```python
from build123d import *

# Parameters (mm, degrees)
SKETCH1_W           = 46
SKETCH1_H           = 160
SKETCH1_R           = 3.05
SKETCH1_R_2         = 4.425
BOSS_EXTRUDE2_DEPTH = 5
SKETCH4_W           = 46
SKETCH4_H           = 160
BOSS_EXTRUDE3_DEPTH = 5
SKETCH5_R           = 16.5
CUT_EXTRUDE2_DEPTH  = 5
SKETCH5_6_R         = 20.5
SKETCH5_6_R_2       = 16.5
BOSS_EXTRUDE5_DEPTH = 10
BOSS_EXTRUDE7_DEPTH = 61.5
SKETCH8_W           = 11.5
SKETCH8_H           = 67.35
SKETCH8_H_2         = 92.65
CUT_EXTRUDE3_DEPTH  = 10
SKETCH10_W          = 11.5
SKETCH10_H          = 115.012630191
CUT_EXTRUDE5_DEPTH  = 10
SKETCH11_R          = 4.425
CUT_EXTRUDE6_DEPTH  = 10
SKETCH12_W          = 11.5
SKETCH12_H          = 11.545
CUT_EXTRUDE7_DEPTH  = 10
SKETCH13_W          = 11.5
SKETCH13_H          = 11.545
CUT_EXTRUDE8_DEPTH  = 10


with BuildPart() as part:
    # Sketch1 → Boss-Extrude2 (new body)
    with BuildSketch(Plane(origin=(0, 0, 0), x_dir=(1, 0, 0), z_dir=(0, 1, 0))):
        with Locations((0, -55)):
            Rectangle(SKETCH1_W, SKETCH1_H)
        with Locations(Location((0, 0, 0), (0, 0, 270))):
            Circle(SKETCH1_R, mode=Mode.SUBTRACT)
        with Locations(Location((0, -113.03, 0), (0, 0, 270))):
            Circle(SKETCH1_R_2, mode=Mode.SUBTRACT)
    extrude(amount=BOSS_EXTRUDE2_DEPTH)



with BuildPart() as body_2:
    # Sketch4 → Boss-Extrude3 (new body)
    with BuildSketch(Plane(origin=(0, 71.5, 0), x_dir=(1, 0, 0), z_dir=(0, 1, 0))):
        with Locations((0, -55)):
            Rectangle(SKETCH4_W, SKETCH4_H)
    extrude(amount=-BOSS_EXTRUDE3_DEPTH)

    # Sketch5 → Cut-Extrude2 (cut)
    with BuildSketch(Plane(origin=(0, 71.5, 0), x_dir=(1, 0, 0), z_dir=(0, 1, 0))):
        with Locations(Location((0, 0, 0), (0, 0, 270))):
            Circle(SKETCH5_R)
    extrude(amount=-CUT_EXTRUDE2_DEPTH, mode=Mode.SUBTRACT)

    # Sketch5<6> → Boss-Extrude5 (add)
    with BuildSketch(Plane(origin=(0, 71.5, 0), x_dir=(1, 0, 0), z_dir=(0, 1, 0))):
        with Locations(Location((0, 0, 0), (0, 0, 90))):
            Circle(SKETCH5_6_R)
        with Locations(Location((0, 0, 0), (0, 0, 270))):
            Circle(SKETCH5_6_R_2, mode=Mode.SUBTRACT)
    extrude(amount=BOSS_EXTRUDE5_DEPTH)


with BuildPart() as part_1:
    add(part.part)

    add(body_2.part)  # Boss-Extrude7 merges body 2
    # Sketch7 → Boss-Extrude7 (add)
    with BuildSketch(Plane(origin=(0, 5, 0), x_dir=(1, 0, 0), z_dir=(0, 1, 0))):
        with BuildLine():
            Line((7.5, -57.65), (-7.5, -57.65))
            Line((-7.5, -57.65), (-7.5, -62.65))
            Line((-7.5, -62.65), (-3, -62.65))
            ThreePointArc((-3, -62.65), (0, -59.65), (3, -62.65))
            Line((3, -62.65), (7.5, -62.65))
            Line((7.5, -62.65), (7.5, -57.65))
        make_face()
        with BuildLine():
            Line((-3, -62.65), (-7.5, -62.65))
            Line((-7.5, -62.65), (-7.5, -67.65))
            Line((-7.5, -67.65), (7.5, -67.65))
            Line((7.5, -67.65), (7.5, -62.65))
            Line((7.5, -62.65), (3, -62.65))
            ThreePointArc((3, -62.65), (0, -65.65), (-3, -62.65))
        make_face()
        with BuildLine():
            ThreePointArc((3, -62.65), (0, -59.65), (-3, -62.65))
            Line((-3, -62.65), (3, -62.65))
        make_face()
        with BuildLine():
            Line((3, -62.65), (-3, -62.65))
            ThreePointArc((-3, -62.65), (0, -65.65), (3, -62.65))
        make_face()
    extrude(amount=BOSS_EXTRUDE7_DEPTH)

    # Sketch8 → Cut-Extrude3 (cut)
    with BuildSketch(Plane(origin=(0, 5, 0), x_dir=(1, 0, 0), z_dir=(0, 1, 0))):
        with Locations((-17.25, -101.325)):
            Rectangle(SKETCH8_W, SKETCH8_H)
        with Locations((-17.25, -21.325)):
            Rectangle(SKETCH8_W, SKETCH8_H_2)
        with Locations((17.25, -101.325)):
            Rectangle(SKETCH8_W, SKETCH8_H)
        with Locations((17.25, -21.325)):
            Rectangle(SKETCH8_W, SKETCH8_H_2)
    extrude(amount=-CUT_EXTRUDE3_DEPTH, mode=Mode.SUBTRACT)

    # Sketch10 → Cut-Extrude5 (cut)
    with BuildSketch(Plane.XZ.offset(-66.5)):
        with Locations((-17.25, 77.493684905)):
            Rectangle(SKETCH10_W, SKETCH10_H)
        with Locations((17.25, 77.493684905)):
            Rectangle(SKETCH10_W, SKETCH10_H)
    extrude(amount=-CUT_EXTRUDE5_DEPTH, mode=Mode.SUBTRACT)

    # Sketch11 → Cut-Extrude6 (cut)
    with BuildSketch(Plane.XZ.offset(-66.5)):
        with Locations(Location((0, 113.03, 0), (0, 0, 90))):
            Circle(SKETCH11_R)
    extrude(amount=-CUT_EXTRUDE6_DEPTH, mode=Mode.SUBTRACT)

    # Sketch12 → Cut-Extrude7 (cut)
    with BuildSketch(Plane(origin=(0, 5, 0), x_dir=(1, 0, 0), z_dir=(0, 1, 0))):
        with Locations((-5.75, -129.2275)):
            Rectangle(SKETCH12_W, SKETCH12_H)
        with Locations((5.75, -129.2275)):
            Rectangle(SKETCH12_W, SKETCH12_H)
    extrude(amount=-CUT_EXTRUDE7_DEPTH, mode=Mode.SUBTRACT)

    # Sketch13 → Cut-Extrude8 (cut)
    with BuildSketch(Plane(origin=(0, 71.5, 0), x_dir=(1, 0, 0), z_dir=(0, 1, 0))):
        with Locations((-5.75, -129.2275)):
            Rectangle(SKETCH13_W, SKETCH13_H)
        with Locations((5.75, -129.2275)):
            Rectangle(SKETCH13_W, SKETCH13_H)
    extrude(amount=-CUT_EXTRUDE8_DEPTH, mode=Mode.SUBTRACT)


solid = part_1.part
```
Geometry check sheet. Reference: the model listing, model coordinates, mm. A direction names the side the tool comes from. Round coordinates to 2 decimals unless told otherwise and drop trailing zeros. Loops run counter-clockwise (first coordinate to the right, second up) from the corner with the lowest first, then second, coordinate; pieces in that order, holes last. Notation, with made-up numbers: (22.5, -31) - (46.5, -31) arc R14 ccw to (46.5, -4) - close; hole circle Ø8 at (-32, 62.25). An arc over 180 degrees is marked (long way). Use a Markdown table: item, result.
Q1. Access from +Z, -Z, +X, -X, +Y, -Y to the whole of each face (thin tool, end or side, straight path). Record for faces 5 (the flat face through (7.5, 35, 63)), 6 (the flat face through (-11.5, 3, 50)), 7 (the flat face through (-7.5, 35, 63)), 8 (the flat face through (0, 35, 57.65)).
Solutions:
| item | result |
|---|---|
| face 5 | +Z, -Z, +X |
| face 6 | +Z, -Z, -X, -Y |
| face 7 | +Z, -Z, -X |
| face 8 | -Z, +X, -X |
Q2. Material ranges on line 1 (Y direction, x = 5, z = 46); line 2 (X direction, y = 1.9, z = 0); line 3 (X direction, y = 2, z = 113), recorded low to high.
Solutions:
| item | result |
|---|---|
| line 1 | y = 0 to 5, 66.5 to 71.5 |
| line 2 | x = -11.5 to -3.05, 3.05 to 11.5 |
| line 3 | x = -11.5 to -4.42, 4.42 to 11.5 |
Q3. Cross-section at B-B on x = 0. State how many separate pieces and enclosed holes the cut face has, plus the area to 3 significant figures.
Solutions:
| item | result |
|---|---|
| separate pieces | 5 |
| enclosed holes | 0 |
| area | 1,900 mm2 |
Q4. Go/stop test with flat-tipped pins: P1, Ø2.5, axis at x = -18, y = 69, coming from the +Z side; P2, Ø4, axis at x = 9, z = 21.5, coming from the +Y side; P3, Ø2, axis at x = 6, z = 28, coming from the -Y side; P4, Ø4, axis at y = 69.5, z = 81.5, coming from the +X side. Record where each tip stops, or that it passes through.
Solutions:
| item | result |
|---|---|
| P1 | stops at z = 19.99 |
| P2 | stops at y = 71.5 |
| P3 | stops at y = 0 |
| P4 | stops at x = 11.5 |
Q5. Draft check along Z on faces 1 (the cylindrical face through (-1.33, 68.96, 117.25)), 2 (the flat face through (11.5, 3, 48)), 3 (the flat face through (0, 2, -25)), 4 (the flat face through (0, 35, 67.65)). Enter one of: released by +Z, released by -Z, zero draft, split by the parting line, or undercut.
Solutions:
| item | result |
|---|---|
| face 1 | undercut |
| face 2 | zero draft |
| face 3 | released by -Z |
| face 4 | released by +Z |
Q6. Cross-section at C-C on z = 14.5. Record the cut outline in (x, y), plus the area to 3 significant figures.
Solutions:
| item | result |
|---|---|
| outline | (-23, 66.5) - (-7.87, 66.5) - (-7.87, 81.5) - (-14.49, 81.5) - (-14.49, 71.5) - (-23, 71.5) - close; (-11.5, 0) - (11.5, 0) - (11.5, 5) - (-11.5, 5) - close; (7.87, 66.5) - (23, 66.5) - (23, 71.5) - (14.49, 71.5) - (14.49, 81.5) - (7.87, 81.5) - close |
| area | 399 mm2 |
Q7. Cross-section at A-A on z = 113.03. Record the cut outline in (x, y) (3 decimals), plus the area to 4 significant figures.
Solutions:
| item | result |
|---|---|
| outline | (-11.5, 0) - (-4.425, 0) - (-4.425, 5) - (-11.5, 5) - close; (-11.5, 66.5) - (-4.425, 66.5) - (-4.425, 71.5) - (-11.5, 71.5) - close; (4.425, 0) - (11.5, 0) - (11.5, 5) - (4.425, 5) - close; (4.425, 66.5) - (11.5, 66.5) - (11.5, 71.5) - (4.425, 71.5) - close |
| area | 141.5 mm2 |
Q8. Cross-section at D-D on z = 61. Record the cut outline in (x, y), plus the area to 3 significant figures.
Solutions:
| item | result |
|---|---|
| outline | (-11.5, 0) - (11.5, 0) - (11.5, 5) - (7.5, 5) - (7.5, 66.5) - (11.5, 66.5) - (11.5, 71.5) - (-11.5, 71.5) - (-11.5, 66.5) - (-7.5, 66.5) - (-7.5, 5) - (-11.5, 5) - close |
| area | 1,150 mm2 |
